Could you check a few things on this model? Use its own coordinates, in mm. A direction names the side the tool comes from. Coordinates: 2 decimals unless noted, no trailing zeros. Loops run counter-clockwise (first coordinate to the right, second up) from the corner with the lowest first, then second, coordinate; pieces in that order, holes last. Notation, with made-up numbers: (52.25, 77) -> (98.25, 77) arc R19 cw to (98.25, 104) -> close; hole circle Ø6 at (66, -5.75). An arc over 180 degrees is marked (long way). One line per question, with ' | ' between items.
```python
from build123d import *

# Parameters (mm, degrees)
SKETCH1_R                         = 6.1976
BOSS_EXTRUDE1_DEPTH               = 15.24
SKETCH2_R                         = 4.7625
CUT_EXTRUDE1_DEPTH                = 0.635
F_1_4_20_TAPPED_HOLE1_D           = 5.1054
F_1_4_20_TAPPED_HOLE1_DEPTH       = 7.62
F_1_4_20_TAPPED_HOLE1_CSINK_D     = 6.3754
F_1_4_20_TAPPED_HOLE1_CSINK_ANGLE = 90
F_1_4_20_TAPPED_HOLE1_TIP         = 1.533816902
FILLET4_R                         = 0.254
SKETCH7_R                         = 0.381
CUT_EXTRUDE2_DEPTH                = 18.580616962
CUT_EXTRUDE2_DEPTH_BACK           = 18.580616962


with BuildPart() as part:
    # Sketch1 → Boss-Extrude1 (new body)
    with BuildSketch(Plane(origin=(0, 0, 0), x_dir=(1, 0, 0), z_dir=(0, 1, 0))):
        with Locations(Location((0, 0, 0), (0, 0, 90))):
            Circle(SKETCH1_R)
    extrude(amount=BOSS_EXTRUDE1_DEPTH)

    # Sketch2 → Cut-Extrude1 (cut)
    with BuildSketch(Plane.XZ):
        with Locations(Location((0, 0, 0), (0, 0, 270))):
            Circle(SKETCH2_R)
    extrude(amount=-CUT_EXTRUDE1_DEPTH, mode=Mode.SUBTRACT)

    # 1/4-20 Tapped Hole1
    with Locations(Plane(origin=(0, 0.635, 0), x_dir=(-1, 0, 0), z_dir=(0, -1, 0))):
        with Locations((0, 0)):
            CounterSinkHole(F_1_4_20_TAPPED_HOLE1_D / 2, F_1_4_20_TAPPED_HOLE1_CSINK_D / 2, depth=F_1_4_20_TAPPED_HOLE1_DEPTH, counter_sink_angle=F_1_4_20_TAPPED_HOLE1_CSINK_ANGLE)
            with Locations((0, 0, -(F_1_4_20_TAPPED_HOLE1_DEPTH + F_1_4_20_TAPPED_HOLE1_TIP / 2))):  # 118° drill point
                Cone(0, F_1_4_20_TAPPED_HOLE1_D / 2, F_1_4_20_TAPPED_HOLE1_TIP, mode=Mode.SUBTRACT)

    # Fillet4
    fillet4_edges = [part.edges().sort_by_distance(p)[0] for p in [
        (0, 0, 6.1976),
    ]]
    fillet(fillet4_edges, radius=FILLET4_R)

    # Sketch7 → Cut-Extrude2 (cut, two sides)
    with BuildSketch(Plane.XY) as cut_extrude2_sk:
        with Locations(Location((0, 0.635, 0), (0, 0, 270))):
            Circle(SKETCH7_R)
        with Locations((0, 8.89)):
            Circle(SKETCH7_R)
    extrude(amount=CUT_EXTRUDE2_DEPTH, mode=Mode.SUBTRACT)
    extrude(cut_extrude2_sk.sketch, amount=-CUT_EXTRUDE2_DEPTH_BACK, mode=Mode.SUBTRACT)


solid = part.part
```
Q1. Imagine slicing it at C-C on y = 10.5. Write out the boundary of the cut face in (x, z).
Values follow:
outline: circle Ø12.4 at (0, 0)
Q2. Imagine slicing it at A-A on y = 8.89. Write out the boundary of the cut face in (x, z).
Values follow:
outline: (-0.38, -6.19) -> (-0.38, -1.45) arc R1.5 cw to (-0.38, 1.45) -> (-0.38, 6.19) arc R6.2 ccw to start; (0.38, -6.19) arc R6.2 ccw to (0.38, 6.19) -> (0.38, 1.45) arc R1.5 cw to (0.38, -1.45) -> close
Q3. For pin 1 (3.5 mm diameter, centred on x = -2.5, z = 0, fed in from -Y) (3 decimals); pin 2 (4.5 mm diameter, centred on x = 0, z = 0, fed in from -Y); pin 3 (2 mm diameter, centred on y = 9.5, z = 1.5, fed in from -X), each with a flat end and sliding along its axis, tell me the tip position at first contact or that it passes through.
Values follow:
pin 1: stops at y = 0.635 | pin 2: stops at y = 8.44 | pin 3: stops at x = -6.18
Q4. Imagine slicing it at B-B on z = -5.25. Give the number of separate pieces and of enclosed holes in the cut face, plus the area to 3 significant figures.
Values follow:
separate pieces: 1 | enclosed holes: 2 | area: 99.4 mm2
Q5. Please list where these lines run through material, in increasing order: L1, parallel to Y at x = 0, z = -5.15; L2, parallel to Y at x = 4, z = 1 (3 decimals); L3, parallel to Z at x = 2, y = 7.5. Write a range as [from, to].
Values follow:
L1: y = [0, 0.25], [1.02, 8.51], [9.27, 15.24] | L2: y = [0.635, 15.24] | L3: z = [-5.87, -1.59], [1.59, 5.87]
Q6. For faces 1 (the face through (-1.9, 7.6, -5.9)), 2 (the face through (-4, 0.635, 0)), which set-ups out of +Z, -Z, +X, -X, +Y, -Y let a thin tool reach every point of the face, with its end or its side?
Values follow:
face 1: +Y, -Y | face 2: -Y
